Autodesk Inventor part; units mm, degrees
ref_plane "YZ Plane" through (0, 0, 0) normal (1, 0, 0) x (0, 1, 0)
ref_plane "XZ Plane" through (0, 0, 0) normal (0, 1, 0) x (-1, 0, 0)
ref_plane "XY Plane" through (0, 0, 0) normal (0, 0, 1) x (1, 0, 0)
ref_plane "Work Plane1" through (0, 0, 0) normal (0, 0, 1) x (1, 0, 0)
sketch "Sketch1" plane through (0, 0, 0) normal (0, 0, 1) x (1, 0, 0)
  circle A0 centre (0, -18.9) radius 1.4
  line L0 (3, -43.9) -> (-3, -43.9)
  line L1 (-5, -41.9) -> (-5, 4.1)
  line L2 (-3, 6.1) -> (3, 6.1)
  line L3 (5, 4.1) -> (5, -41.9)
  line L4 (5, -43.9) -> (-5, 6.1) construction
  line L5 (-5, -43.9) -> (5, 6.1) construction
  arc A1 (-5, -41.9) -> (-3, -43.9) centre (-3, -41.9) ccw
  arc A2 (3, -43.9) -> (5, -41.9) centre (3, -41.9) ccw
  arc A3 (5, 4.1) -> (3, 6.1) centre (3, 4.1) ccw
  arc A4 (-3, 6.1) -> (-5, 4.1) centre (-3, 4.1) ccw
  point P0 (0, 0)
  dimension "d0" = 10
  dimension "d1" = 50
  dimension "d2" = 2
extrude "Extrusion1" add sketch "Sketch1" along normal blind 3
properties part number "20_Cube_4_insert_xy_levelarm_2"
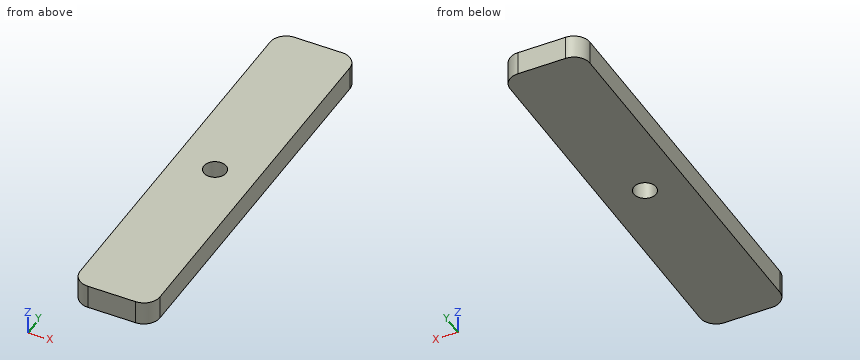
Could you check a few things on this model? Use its own coordinates, in mm. Give positions to 0.01 mm unless a question says otherwise; leave off trailing zeros. Order: outer loops, then holes, each group sorted by start corner. A loop starts at its lowest first (then second) coordinate and runs counter-clockwise, first axis right, second up.
Q1. Suppose I cut it at C-C, the plane z = 0.7. Write out the boundary of the cut face in (x, y), and give its area (3 significant figures).
Q2. Suppose I cut it at A-A, the plane y = -18.9. Write out the boundary of the cut face in (x, z), and give its area (3 significant figures).
Q3. I'm going to push a flat-ended pin straight in: P1, Ø3, axis at x = -0.5, y = -27, coming from the -Z side. Where does the tip first touch, or does it pass through?
Q4. If I drill on line 1 along Y through (x, z) = (0, 1.2); line 2 along Y through (x, z) = (-1, 1.35); line 3 along Y through (x, z) = (4.5, 0.9), over which ranges is the centre line in solid material (lowest first)?
Q5. Suppose I cut it at B-B, the plane x = 0. Write out the boundary of the cut face in (y, z).
Q6. Suppose I cut it at D-D, the plane x = 4.5. Write out the boundary of the cut face in (y, z).
Solution:
1. outline: (-5, -41.9) arc R2 ccw to (-3, -43.9) - (3, -43.9) arc R2 ccw to (5, -41.9) - (5, 4.1) arc R2 ccw to (3, 6.1) - (-3, 6.1) arc R2 ccw to (-5, 4.1) - close; hole circle Ø2.8 at (0, -18.9)
1. area: 490 mm2
2. outline: (-5, 0) - (-1.4, 0) - (-1.4, 3) - (-5, 3) - close; (1.4, 0) - (5, 0) - (5, 3) - (1.4, 3) - close
2. area: 21.6 mm2
3. P1: stops at z = 0
4. line 1: y = -43.9 to -20.3, -17.5 to 6.1
4. line 2: y = -43.9 to -19.88, -17.92 to 6.1
4. line 3: y = -43.22 to 5.42
5. outline: (-43.9, 0) - (-20.3, 0) - (-20.3, 3) - (-43.9, 3) - close; (-17.5, 0) - (6.1, 0) - (6.1, 3) - (-17.5, 3) - close
6. outline: (-43.22, 0) - (5.42, 0) - (5.42, 3) - (-43.22, 3) - close
